from build123d import *
from build123d.topology import SkipClean

# Parameters (mm, degrees)
BOSS_EXTRUDE1_DEPTH           = 3
BOSS_EXTRUDE2_START           = -1.75
SKETCH1_3_R                   = 11
BOSS_EXTRUDE2_DEPTH           = 1.75
SKETCH2_R                     = 1.75
CUT_EXTRUDE1_DEPTH            = 4.75
SKETCH2_3_R                   = 3
CUT_EXTRUDE2_DEPTH            = 1.75
BOSS_EXTRUDE3_START           = -1.225
SKETCH1_4_R                   = 11
BOSS_EXTRUDE3_DEPTH           = 1.225
SKETCH3_R                     = 1.6
CUT_EXTRUDE3_DEPTH            = 4.225
SKETCH3_3_R                   = 3
SKETCH3_3_R_2                 = 1.6
CUT_EXTRUDE4_DEPTH            = 1.225
BODY_MOVE_COPY1_DEPTH         = 3
BODY_MOVE_COPY1_START         = 1.75
BODY_MOVE_COPY1_2_OUTLINE_R   = 11
BODY_MOVE_COPY1_2_OUTLINE_R_2 = 1.6
BODY_MOVE_COPY1_2_OUTLINE_R_3 = 3
BODY_MOVE_COPY1_2_DEPTH       = 1.25
BODY_MOVE_COPY1_START_2       = 1.225
BODY_MOVE_COPY1_3_OUTLINE_R   = 11
BODY_MOVE_COPY1_3_OUTLINE_R_2 = 1.6
BODY_MOVE_COPY1_3_DEPTH       = 0.525
BODY_MOVE_COPY1_START_3       = -1.75
BODY_MOVE_COPY1_4_OUTLINE_R   = 3
BODY_MOVE_COPY1_4_OUTLINE_R_2 = 1.75
BODY_MOVE_COPY1_4_DEPTH       = 0.5
BODY_MOVE_COPY1_START_4       = -3
BODY_MOVE_COPY1_5_OUTLINE_R   = 3
BODY_MOVE_COPY1_5_DEPTH       = 3
BODY_MOVE_COPY1_START_5       = -1.775
BODY_MOVE_COPY1_6_OUTLINE_R   = 3
BODY_MOVE_COPY1_6_OUTLINE_R_2 = 1.6
BODY_MOVE_COPY1_6_DEPTH       = 0.55
BODY_MOVE_COPY1_START_6       = 1.25
BODY_MOVE_COPY1_7_OUTLINE_R   = 3
BODY_MOVE_COPY1_7_OUTLINE_R_2 = 1.75
BODY_MOVE_COPY1_7_DEPTH       = 0.5


# Read off the part's stored shape, not the designer's step: Body-Move/Copy1
with BuildPart() as part:
    # Sketch1 → Boss-Extrude1 (new body)
    with BuildSketch(Plane.XY):
        with BuildLine():
            Line((-11, 30), (-11, -30))
            ThreePointArc((-11, -30), (0, -41), (11, -30))
            Line((11, -30), (11, 30))
            ThreePointArc((11, 30), (0, 41), (-11, 30))
        make_face()
        with BuildLine():
            ThreePointArc((5, -19.643842411), (0, -18.5), (-5, -19.643842411))
            Line((-5, -19.643842411), (-5, 19.643842411))
            ThreePointArc((-5, 19.643842411), (0, 18.5), (5, 19.643842411))
            Line((5, 19.643842411), (5, -19.643842411))
        make_face(mode=Mode.SUBTRACT)
    extrude(amount=BOSS_EXTRUDE1_DEPTH)

    # Sketch1<3> → Boss-Extrude2 (add)
    with BuildSketch(Plane.XY.offset(BOSS_EXTRUDE2_START)):
        with Locations((0, 30)):
            Circle(SKETCH1_3_R)
    extrude(amount=BOSS_EXTRUDE2_DEPTH)

    # Sketch2 → Cut-Extrude1 (cut)
    with BuildSketch(Plane.XY.offset(3)):
        with Locations((0, 30)):
            Circle(SKETCH2_R)
    extrude(amount=-CUT_EXTRUDE1_DEPTH, mode=Mode.SUBTRACT)

    # Sketch2<3> → Cut-Extrude2 (cut)
    with BuildSketch(Plane.XY.offset(3)):
        with Locations((0, 30)):
            Circle(SKETCH2_3_R)
    extrude(amount=-CUT_EXTRUDE2_DEPTH, mode=Mode.SUBTRACT)

    # Sketch1<4> → Boss-Extrude3 (add)
    with SkipClean():  # the faces are left unmerged after this step: merging them gives an invalid solid
        with BuildSketch(Plane.XY.offset(BOSS_EXTRUDE3_START)):
            with Locations((0, -30)):
                Circle(SKETCH1_4_R)
        extrude(amount=BOSS_EXTRUDE3_DEPTH)

    # Sketch3 → Cut-Extrude3 (cut)
    with SkipClean():  # the faces are left unmerged after this step: merging them gives an invalid solid
        with BuildSketch(Plane.XY.offset(3)):
            with Locations((0, -30)):
                Circle(SKETCH3_R)
        extrude(amount=-CUT_EXTRUDE3_DEPTH, mode=Mode.SUBTRACT)

    # Sketch3<3> → Cut-Extrude4 (cut)
    with SkipClean():  # the faces are left unmerged after this step: merging them gives an invalid solid
        with BuildSketch(Plane.XY.offset(3)):
            with Locations((0, -30)):
                Circle(SKETCH3_3_R)
            with Locations((0, -30)):
                Circle(SKETCH3_3_R_2, mode=Mode.SUBTRACT)
        extrude(amount=-CUT_EXTRUDE4_DEPTH, mode=Mode.SUBTRACT)

    # Body-Move/Copy1 outline → Body-Move/Copy1 (cut)
    with SkipClean():  # the faces are left unmerged after this step: merging them gives an invalid solid
        with BuildSketch(Plane.XY):
            with BuildLine():
                Line((-11, 30), (-11, -30))
                ThreePointArc((-11, -30), (0, -19), (11, -30))
                Line((11, -30), (11, 30))
                ThreePointArc((11, 30), (0, 19), (-11, 30))
            make_face()
            with BuildLine():
                Line((-5, -19.643842411), (-5, 19.643842411))
                ThreePointArc((-5, 19.643842411), (0, 18.5), (5, 19.643842411))
                Line((5, 19.643842411), (5, -19.643842411))
                ThreePointArc((5, -19.643842411), (0, -18.5), (-5, -19.643842411))
            make_face(mode=Mode.SUBTRACT)
        extrude(amount=BODY_MOVE_COPY1_DEPTH, mode=Mode.SUBTRACT)

    # Body-Move_Copy1 2 outline → Body-Move_Copy1 2 (cut)
    # profile 1 of 2: a face of its own
    with SkipClean():  # the faces are left unmerged after this step: merging them gives an invalid solid
        with BuildSketch(Plane.XY.offset(BODY_MOVE_COPY1_START)):
            with Locations((0, -30)):
                Circle(BODY_MOVE_COPY1_2_OUTLINE_R)
            with Locations((0, -30)):
                Circle(BODY_MOVE_COPY1_2_OUTLINE_R_2, mode=Mode.SUBTRACT)
        # profile 2 of 2: a face of its own
        with BuildSketch(Plane.XY.offset(BODY_MOVE_COPY1_START)):
            with Locations((0, 30)):
                Circle(BODY_MOVE_COPY1_2_OUTLINE_R)
            with Locations((0, 30)):
                Circle(BODY_MOVE_COPY1_2_OUTLINE_R_3, mode=Mode.SUBTRACT)
        extrude(amount=BODY_MOVE_COPY1_2_DEPTH, mode=Mode.SUBTRACT)

    # Body-Move_Copy1 3 outline → Body-Move_Copy1 3 (cut)
    with SkipClean():  # the faces are left unmerged after this step: merging them gives an invalid solid
        with BuildSketch(Plane.XY.offset(BODY_MOVE_COPY1_START_2)):
            with Locations((0, -30)):
                Circle(BODY_MOVE_COPY1_3_OUTLINE_R)
            with Locations((0, -30)):
                Circle(BODY_MOVE_COPY1_3_OUTLINE_R_2, mode=Mode.SUBTRACT)
        extrude(amount=BODY_MOVE_COPY1_3_DEPTH, mode=Mode.SUBTRACT)

    # Body-Move_Copy1 4 outline → Body-Move_Copy1 4 (cut)
    with SkipClean():  # the faces are left unmerged after this step: merging them gives an invalid solid
        with BuildSketch(Plane.XY.offset(BODY_MOVE_COPY1_START_3)):
            with Locations((0, 30)):
                Circle(BODY_MOVE_COPY1_4_OUTLINE_R)
            with Locations((0, 30)):
                Circle(BODY_MOVE_COPY1_4_OUTLINE_R_2, mode=Mode.SUBTRACT)
        extrude(amount=BODY_MOVE_COPY1_4_DEPTH, mode=Mode.SUBTRACT)

    # Body-Move_Copy1 5 outline → Body-Move_Copy1 5 (add)
    with BuildSketch(Plane.XY.offset(BODY_MOVE_COPY1_START_4)):
        with BuildLine():
            Line((-11, 30), (-11, -30))
            ThreePointArc((-11, -30), (0, -41), (11, -30))
            Line((11, -30), (11, 30))
            ThreePointArc((11, 30), (0, 41), (-11, 30))
        make_face()
        with BuildLine():
            Line((-5, -19.643842411), (-5, 19.643842411))
            ThreePointArc((-5, 19.643842411), (0, 18.5), (5, 19.643842411))
            Line((5, 19.643842411), (5, -19.643842411))
            ThreePointArc((5, -19.643842411), (0, -18.5), (-5, -19.643842411))
        make_face(mode=Mode.SUBTRACT)
        with Locations((0, 30)):
            Circle(BODY_MOVE_COPY1_5_OUTLINE_R, mode=Mode.SUBTRACT)
        with Locations((0, -30)):
            Circle(BODY_MOVE_COPY1_5_OUTLINE_R, mode=Mode.SUBTRACT)
    extrude(amount=BODY_MOVE_COPY1_5_DEPTH)

    # Body-Move_Copy1 6 outline → Body-Move_Copy1 6 (add)
    with SkipClean():  # the faces are left unmerged after this step: merging them gives an invalid solid
        with BuildSketch(Plane.XY.offset(BODY_MOVE_COPY1_START_5)):
            with Locations((0, -30)):
                Circle(BODY_MOVE_COPY1_6_OUTLINE_R)
            with Locations((0, -30)):
                Circle(BODY_MOVE_COPY1_6_OUTLINE_R_2, mode=Mode.SUBTRACT)
        extrude(amount=BODY_MOVE_COPY1_6_DEPTH)

    # Body-Move_Copy1 7 outline → Body-Move_Copy1 7 (add)
    with BuildSketch(Plane.XY.offset(BODY_MOVE_COPY1_START_6)):
        with Locations((0, 30)):
            Circle(BODY_MOVE_COPY1_7_OUTLINE_R)
        with Locations((0, 30)):
            Circle(BODY_MOVE_COPY1_7_OUTLINE_R_2, mode=Mode.SUBTRACT)
    extrude(amount=BODY_MOVE_COPY1_7_DEPTH)


solid = part.part
Work out the finished part from the listing and answer in its coordinate system (mm). A direction names the side the tool comes from. Give positions to 0.01 mm unless a question says otherwise; leave off trailing zeros. Loops run counter-clockwise (first coordinate to the right, second up) from the corner with the lowest first, then second, coordinate; pieces in that order, holes last. Notation, with made-up numbers: (22, 11) - (48, 11) arc R30 ccw to (48, 49) - close; hole circle Ø10 at (82.25, -15). An arc over 180 degrees is marked (long way). Answer in a Markdown table with one row per item. Add a question column.
Q1. A tool of negligible diameter and unlimited length cuts with its end or side. For faces 3 (the flat face through (0, 28, -1.25)), 4 (the flat face through (-5, 0, -2)), 5 (the flat face through (0, -32, 1.225)), from which of +Z, -Z, +X, -X, +Y, -Y can it reach the whole face along a straight path? Write none if from no direction.
Q2. Consider line 1 along Y through (x, z) = (0, 1.6); line 2 along Y through (x, z) = (-0.75, -1.45); line 3 along X through (y, z) = (17.5, -1.2). Determine where each line is inside the solid, lowest interval first.
Q3. Each of these flat-tipped pins is pushed along its axis until it touches: P1, Ø6.5, axis at x = 2, y = 9, coming from the +Z side; P2, Ø6, axis at x = -4.5, y = -18, coming from the +Z side (3 decimals); P3, Ø5.5, axis at x = 0, y = -30, coming from the -Z side (3 decimals). Where does it stop, or does it pass through?
Q4. The part is cut by section C-C (x = 8.25). Determine the outline of the cut face in (y, z) (3 decimals).
Q5. The part is cut by section B-B (y = -10). Determine the outline of the cut face in (x, z), and give its area (3 significant figures).
Q6. The part is cut by section A-A (x = 0). Determine the outline of the cut face in (y, z) (3 decimals).
Q7. Determine the mould class of faces 1 (the flat face through (5, 0, -2)), 2 (the flat face through (-7, 1, -3)) for opening direction Y: released by +Y, released by -Y, zero draft, split by the parting line, or undercut.
Q8. The part is cut by section D-D (y = 34.5). Determine the outline of the cut face in (x, z).
Solution:
| question | item | result |
|---|---|---|
| 1 | face 3 | -Z |
| 1 | face 4 | +Z, -Z |
| 1 | face 5 | +Z, +X, -X, -Y |
| 2 | line 1 | y = 19 to 28.25, 31.75 to 41 |
| 2 | line 2 | y = -40.97 to -31.41, -28.59 to -18.52, 18.52 to 27.1, 32.9 to 40.97 |
| 2 | line 3 | x = -11 to -5, 5 to 11 |
| 3 | P1 | stops at z = 0 |
| 3 | P2 | stops at z = 1.225 |
| 3 | P3 | stops at z = -1.775 |
| 4 | outline | (-37.276, -3) - (37.276, -3) - (37.276, 1.75) - (22.724, 1.75) - (22.724, 0) - (-22.724, 0) - (-22.724, 1.225) - (-37.276, 1.225) - close |
| 5 | outline | (-11, -3) - (-5, -3) - (-5, 0) - (-11, 0) - close; (5, -3) - (11, -3) - (11, 0) - (5, 0) - close |
| 5 | area | 36.0 mm² |
| 6 | outline | (-41, -3) - (-33, -3) - (-33, -1.775) - (-31.6, -1.775) - (-31.6, 1.225) - (-41, 1.225) - close; (-28.4, -1.775) - (-27, -1.775) - (-27, -3) - (-18.5, -3) - (-18.5, 0) - (-19, 0) - (-19, 1.225) - (-28.4, 1.225) - close; (18.5, -3) - (27, -3) - (27, -1.25) - (28.25, -1.25) - (28.25, 1.75) - (19, 1.75) - (19, 0) - (18.5, 0) - close; (31.75, -1.25) - (33, -1.25) - (33, -3) - (41, -3) - (41, 1.75) - (31.75, 1.75) - close |
| 7 | face 1 | undercut |
| 7 | face 2 | zero draft |
| 8 | outline | (-10.04, -3) - (10.04, -3) - (10.04, 1.75) - (-10.04, 1.75) - close |
